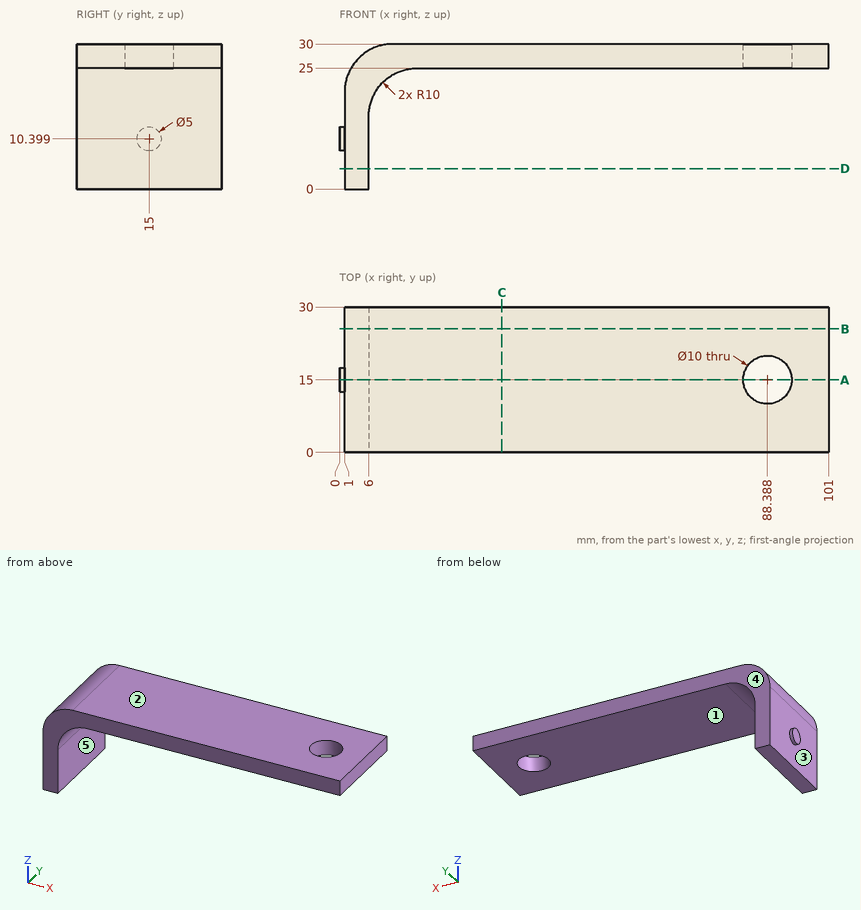
The drawing under review shows one solid part. Ordinate dimensions are in mm from its lowest x, y, z. A direction names the side the tool comes from. Give positions to 0.01 mm unless a question says otherwise; leave off trailing zeros. Write each loop counter-clockwise with the first axis right and the second up, starting at its lowest first coordinate (ties: lowest second). Pieces come first, ordered by that corner, then holes. Notation, with made-up numbers: (32, -28) -> (88, -28) arc R28 ccw to (88, 1) -> close; hole circle Ø6 at (-19.75, 72). An arc over 180 degrees is marked (long way). Put each result on its own line as item: value.
(1) We need section A-A, the plane y = 15. Give the boundary of the cut face in (x, z), and give its area (3 significant figures).
Results are:
outline: (0, 7.9) -> (1, 7.9) -> (1, 0) -> (6, 0) -> (6, 15) arc R10 cw to (16, 25) -> (83.39, 25) -> (83.39, 30) -> (11, 30) arc R10 ccw to (1, 20) -> (1, 12.9) -> (0, 12.9) -> close; (93.39, 25) -> (101, 25) -> (101, 30) -> (93.39, 30) -> close
area: 580 mm²
(2) To check wall thickness, follow probe 1 along Z at (x, y) = (22.5, 11); probe 2 along X at (y, z) = (9, 3); probe 3 along X at (y, z) = (18.75, 27) (1 decimal). State the ranges of each line that lie inside material, in increasing order. Write a range as from..to.
Results are:
probe 1: 25..30
probe 2: 1..6
probe 3: 3.9..85.1, 91.7..101
(3) Tool access review of the marked faces 4 and 5: name each direction out of +Z, -Z, +X, -X, +Y, -Y from which nothing blocks a thin tool from reaching the whole face with its end or side.
Results are:
face 4: +Z, -Z, +X, -X, +Y
face 5: -Z, +X, +Y, -Y
(4) The part is to be moulded in two halves that separate along Z. For the marked faces 1, 2 and 3, say which applies: pulls with the +Z half, pulls with the -Z half, needs draft (parallel to the pull), parting line crosses it, or undercut.
Results are:
face 1: pulls with the -Z half
face 2: pulls with the +Z half
face 3: needs draft
(5) We need section B-B, the plane y = 25.5. Give the boundary of the cut face in (x, z).
Results are:
outline: (1, 0) -> (6, 0) -> (6, 15) arc R10 cw to (16, 25) -> (101, 25) -> (101, 30) -> (11, 30) arc R10 ccw to (1, 20) -> close
(6) For pin 1 Ø12 at (y, z) = (19.5, 7) entering from +X; pin 2 Ø3 at (x, y) = (48, 25.5) entering from -Z; pin 3 Ø5 at (y, z) = (7, 19.5) entering from +X, all flat-tipped, find the tip position at first contact; note any pin that passes through.
Results are:
pin 1: x = 6
pin 2: z = 25
pin 3: x = 8.86
(7) We need section D-D, the plane z = 4.25. Give the boundary of the cut face in (x, y), and give its area (3 significant figures).
Results are:
outline: (1, 0) -> (6, 0) -> (6, 30) -> (1, 30) -> close
area: 150 mm²
(8) We need section C-C, the plane x = 33.5. Give the boundary of the cut face in (y, z), and give its area (3 significant figures).
Results are:
outline: (0, 25) -> (30, 25) -> (30, 30) -> (0, 30) -> close
area: 150 mm²
